```python
from build123d import *

# Parameters (mm, degrees)
SKETCH_1_W          = 16
SKETCH_1_H          = 16
SKETCH_1_W_2        = 10
SKETCH_1_H_2        = 10
EXTRUDE_1_DEPTH     = 20
CUT_EXTRUDE_1_DEPTH = 16


with BuildPart() as part:
    # 草图1 → 凸台-拉伸1 (new body)
    with BuildSketch(Plane.XY):
        with Locations((8, 8)):
            Rectangle(SKETCH_1_W, SKETCH_1_H)
        with Locations((8, 8)):
            Rectangle(SKETCH_1_W_2, SKETCH_1_H_2, mode=Mode.SUBTRACT)
    extrude(amount=EXTRUDE_1_DEPTH)

    # 草图2 → 切除-拉伸1 (cut)
    with BuildSketch(Plane(origin=(16, 0, 0), x_dir=(0, 0, -1), z_dir=(1, 0, 0))):
        with BuildLine():
            Line((-4, 9), (-16, 9))
            ThreePointArc((-16, 9), (-15.292893219, 8.707106781), (-15, 8))
            ThreePointArc((-15, 8), (-15.292893219, 7.292893219), (-16, 7))
            Line((-16, 7), (-4, 7))
            ThreePointArc((-4, 7), (-5, 8), (-4, 9))
        make_face()
        with BuildLine():
            ThreePointArc((-3, 8), (-3.292893219, 8.707106781), (-4, 9))
            Line((-4, 9), (-4, 7))
            ThreePointArc((-4, 7), (-3.292893219, 7.292893219), (-3, 8))
        make_face()
        with BuildLine():
            Line((-4, 7), (-4, 9))
            ThreePointArc((-4, 9), (-5, 8), (-4, 7))
        make_face()
        with BuildLine():
            ThreePointArc((-15, 8), (-15.292893219, 8.707106781), (-16, 9))
            Line((-16, 9), (-16, 7))
            ThreePointArc((-16, 7), (-15.292893219, 7.292893219), (-15, 8))
        make_face()
        with BuildLine():
            Line((-16, 7), (-16, 9))
            ThreePointArc((-16, 9), (-17, 8), (-16, 7))
        make_face()
    extrude(amount=-CUT_EXTRUDE_1_DEPTH, mode=Mode.SUBTRACT)


solid = part.part
```
Work out the finished part from the listing and answer in its coordinate system (mm). A direction names the side the tool comes from. Give positions to 0.01 mm unless a question says otherwise; leave off trailing zeros. Loops run counter-clockwise (first coordinate to the right, second up) from the corner with the lowest first, then second, coordinate; pieces in that order, holes last. Notation, with made-up numbers: M -36.75,89 L -8.75,89 A21 cw -8.75,110 Z; hole C 54.25,-23 d9. An arc over 180 degrees is marked long. One line per item, written item: value. Start each with the question number.
1. Find the intervals of material crossed by probe 1 along Y at (x, z) = (3.75, 15.75); probe 2 along Y at (x, z) = (2.75, 9), in increasing order.
2. Which of the six approach directions +Z, -Z, +X, -X, +Y, -Y give full straight-line access (tool end or side, diameter ignored) to faces 1 (the face through (15, 8, 17)), 2 (the face through (16, 10, 10)), 3 (the face through (3, 6.8, 9.9))?
3. Find section B-B (z = 1.5). Give the vertices of the cut face in (x, y), and give its area (3 significant figures).
4. Find section C-C (y = 9.5). Give the vertices of the cut face in (x, z).
5. Find section A-A (z = 9.25). Give the vertices of the cut face in (x, y), and give its area (3 significant figures).
6. Determine the mould class of faces 4 (the face through (8, 16, 10)), 5 (the face through (8, 3, 10)), 6 (the face through (15, 9, 10)), 7 (the face through (13.2, 8.1, 20)) for opening direction Y: released by +Y, released by -Y, zero draft, split by the parting line, or undercut.
Reported:
1. probe 1: y = 0 to 3, 13 to 16
1. probe 2: y = 0 to 7, 9 to 16
2. face 1: +X, -X
2. face 2: +Z, -Z, +X, +Y, -Y
2. face 3: +Z, -Z
3. outline: M 0,0 L 16,0 L 16,16 L 0,16 Z; hole M 3,3 L 13,3 L 13,13 L 3,13 Z
3. area: 156 mm²
4. outline: M 0,0 L 3,0 L 3,20 L 0,20 Z; M 13,0 L 16,0 L 16,20 L 13,20 Z
5. outline: M 0,0 L 16,0 L 16,7 L 13,7 L 13,3 L 3,3 L 3,7 L 0,7 Z; M 0,9 L 3,9 L 3,13 L 13,13 L 13,9 L 16,9 L 16,16 L 0,16 Z
5. area: 144 mm²
6. face 4: released by +Y
6. face 5: undercut
6. face 6: undercut
6. face 7: zero draft
